Could you check a few things on this model? Use its own coordinates, in mm. A direction names the side the tool comes from. Round coordinates to 2 decimals unless told otherwise and drop trailing zeros. Loops run counter-clockwise (first coordinate to the right, second up) from the corner with the lowest first, then second, coordinate; pieces in that order, holes last. Notation, with made-up numbers: (-12, -15.75) -> (19, -15.75) arc R3 cw to (19, -11.75) -> close; hole circle Ø5 at (75, -16). An arc over 180 degrees is marked (long way). One line per item, written item: value.
```python
from build123d import *

# Parameters (mm, degrees)
SKETCH1_W           = 10
SKETCH1_H           = 2.5
BOSS_EXTRUDE1_DEPTH = 15
SKETCH2_R           = 1.5
CUT_EXTRUDE1_DEPTH  = 15
SKETCH3_W           = 10
SKETCH3_H           = 5
BOSS_EXTRUDE2_DEPTH = 10
SKETCH4_W           = 10
SKETCH4_H           = 5
BOSS_EXTRUDE3_DEPTH = 10


with BuildPart() as part:
    # Sketch1 → Boss-Extrude1 (new body)
    with BuildSketch(Plane.XY):
        with Locations((5, -1.25)):
            Rectangle(SKETCH1_W, SKETCH1_H)
    extrude(amount=BOSS_EXTRUDE1_DEPTH)

    # Sketch2 → Cut-Extrude1 (cut)
    with BuildSketch(Plane(origin=(0, 0, 0), x_dir=(1, 0, 0), z_dir=(0, 1, 0))):
        with Locations(Location((5, -12, 0), (0, 0, 270))):
            Circle(SKETCH2_R)
        with Locations(Location((5, -8, 0), (0, 0, 270))):
            Circle(SKETCH2_R)
    extrude(amount=-CUT_EXTRUDE1_DEPTH, mode=Mode.SUBTRACT)

    # Sketch3 → Boss-Extrude2 (add)
    with BuildSketch(Plane(origin=(0, 0, 0), x_dir=(-1, 0, 0), z_dir=(0, 0, -1))):
        with Locations((-5, 0)):
            Rectangle(SKETCH3_W, SKETCH3_H)
    extrude(amount=BOSS_EXTRUDE2_DEPTH)

    # Sketch4 → Boss-Extrude3 (add)
    with BuildSketch(Plane(origin=(0, 2.5, 0), x_dir=(1, 0, 0), z_dir=(0, 1, 0))):
        with Locations((5, 7.5)):
            Rectangle(SKETCH4_W, SKETCH4_H)
    extrude(amount=BOSS_EXTRUDE3_DEPTH)


solid = part.part
```
(1) Imagine slicing it at B-B on z = 12. Write out the boundary of the cut face in (x, y), then the cut area to 3 significant figures.
Results below:
outline: (0, -2.5) -> (3.5, -2.5) -> (3.5, 0) -> (0, 0) -> close; (6.5, -2.5) -> (10, -2.5) -> (10, 0) -> (6.5, 0) -> close
area: 17.5 mm²
(2) Imagine slicing it at C-C on x = 3.75. Write out the boundary of the cut face in (y, z), then the cut area to 3 significant figures.
Results below:
outline: (-2.5, -10) -> (12.5, -10) -> (12.5, -5) -> (2.5, -5) -> (2.5, 0) -> (0, 0) -> (0, 7.17) -> (-2.5, 7.17) -> close; (-2.5, 8.83) -> (0, 8.83) -> (0, 11.17) -> (-2.5, 11.17) -> close; (-2.5, 12.83) -> (0, 12.83) -> (0, 15) -> (-2.5, 15) -> close
area: 129 mm²
(3) We'd pull the mould along X, two halves only. Please class faces 1 (the face through (5.07, -1.23, 6.5)), 2 (the face through (0, 2, -3)), 3 (the face through (5, 12.5, -8)), 4 (the face through (5.07, -1.23, 10.5)): +X half, -X half, draft (parallel to the pull), parting line (faces both ways), or undercut.
Results below:
face 1: undercut
face 2: -X half
face 3: draft
face 4: undercut
(4) Please list where these lines run through material, in increasing order: L1, parallel to X at y = -1.5, z = 8; L2, parallel to Z at x = 6.5, y = 6.75; L3, parallel to Y at x = 3.5, z = 7.25.
Results below:
L1: x = 0 to 3.5, 6.5 to 10
L2: z = -10 to -5
L3: y = -2.5 to 0
(5) Imagine slicing it at A-A on x = 5. Write out the boundary of the cut face in (y, z), then the cut area to 4 significant figures.
Results below:
outline: (-2.5, -10) -> (12.5, -10) -> (12.5, -5) -> (2.5, -5) -> (2.5, 0) -> (0, 0) -> (0, 6.5) -> (-2.5, 6.5) -> close; (-2.5, 9.5) -> (0, 9.5) -> (0, 10.5) -> (-2.5, 10.5) -> close; (-2.5, 13.5) -> (0, 13.5) -> (0, 15) -> (-2.5, 15) -> close
area: 122.5 mm²
(6) For pin 1 Ø3 at (x, y) = (6, 8.5) entering from +Z; pin 2 Ø0.8 at (x, y) = (3.5, 1) entering from +Z; pin 3 Ø1.5 at (x, z) = (5, -2.5) entering from +Y, each with a flat end and sliding along its axis, tell me the tip position at first contact or that it passes through.
Results below:
pin 1: stops at z = -5
pin 2: stops at z = 0
pin 3: stops at y = 2.5
(7) Imagine slicing it at D-D on y = 5.25. Write out the boundary of the cut face in (x, z), then the cut area to 3 significant figures.
Results below:
outline: (0, -10) -> (10, -10) -> (10, -5) -> (0, -5) -> close
area: 50.0 mm²
(8) On a 3-axis mill with a long thin cutter (end or side, diameter ignored), from which of +Z, -Z, +X, -X, +Y, -Y can I reach the whole of each face in a straight line? I mean faces 5 (the face through (5, 2.5, -2)), 6 (the face through (5, -2.5, 3)). Say none if no direction works.
Results below:
face 5: +Z, +X, -X, +Y
face 6: +Z, -Z, +X, -X, -Y
